Input: part model. Units: mm. Frame: model coordinates. A direction names the side the tool comes from. Coordinates: 2 decimals unless noted, no trailing zeros. Write each loop counter-clockwise with the first axis right and the second up, starting at its lowest first coordinate (ties: lowest second). Pieces come first, ordered by that corner, then holes. Notation, with made-up numbers: (81.5, 50) - (122.5, 50) arc R26 cw to (122.5, 68) - close; hole circle Ø1 at (40, 47.25). An arc over 180 degrees is marked (long way). Use a Markdown table: item, result. Add a question column.
Q1. Section query B-B (y = 0). Return the cut outline in (x, z).
Q2. Section query C-C (z = 17.7). Return the cut outline in (x, y).
Q3. Set-up query: faces 4 (the face through (36.198, 11.399, 80.98)), 5 (the face through (0.22, 41.258, 79.855)). Return all of +Z, -Z, +X, -X, +Y, -Y with unobstructed straight access to the full face (end or side cutting, diameter ignored); none if empty.
Q4. Material intervals for probe 1 along Z at (x, y) = (0, 40); probe 2 along Z at (x, y) = (7.5, -33.5); probe 3 along Y at (x, z) = (0, 62), sorted ascending. Write a range as from..to.
Q5. Mould query, pull axis X, two halves, no side actions, for faces 1 (the face through (-24, -30, 150)), 2 (the face through (0.22, -41.361, 79.855)), 3 (the face through (20.765, -39.923, 73.95)). Classes: released by +X, released by -X, zero draft, split by the parting line, or undercut.
Q6. Section query D-D (x = -16.5). Return the cut outline in (y, z).
Q7. Pin query (flat end, axial travel): P1, Ø3, axis at y = -16.5, z = 38.5, coming from the +X side; P2, Ø1.5, axis at y = -19.5, z = 58, coming from the +X side; P3, Ø5, axis at x = -20.5, z = 109.5, coming from the +Y side. Return the tip coordinate at first contact, or that it passes through.
Q8. Section query A-A (x = 0). Return the cut outline in (y, z), then the cut area to 4 significant figures.
from build123d import *

# Parameters (mm, degrees)
SKETCH1_R               = 45
BOSS_EXTRUDE1_DEPTH     = 150
SKETCH2_R               = 31.85
CUT_EXTRUDE1_DEPTH      = 163.941707368
SKETCH3_R               = 37.95
CUT_EXTRUDE2_DEPTH      = 140
CUT_EXTRUDE5_DEPTH      = 163.941707368
CUT_EXTRUDE5_DEPTH_BACK = 163.941707368
SKETCH8_R               = 5


with BuildPart() as part:
    # Sketch1 → Boss-Extrude1 (new body)
    with BuildSketch(Plane.XY):
        Circle(SKETCH1_R)
    extrude(amount=BOSS_EXTRUDE1_DEPTH)

    # Sketch2 → Cut-Extrude1 (cut, through all)
    with BuildSketch(Plane.XY.offset(150)):
        Circle(SKETCH2_R)
    extrude(amount=-CUT_EXTRUDE1_DEPTH, mode=Mode.SUBTRACT)

    # Sketch3 → Cut-Extrude2 (cut)
    with BuildSketch(Plane.XY.offset(150)):
        Circle(SKETCH3_R)
    extrude(amount=-CUT_EXTRUDE2_DEPTH, mode=Mode.SUBTRACT)

    # Sketch8 → Cut-Extrude5 (cut, two sides: drawn at the far end of the back side and taken through both)
    with BuildSketch(Plane(origin=(0, 0, 0), x_dir=(1, 0, 0), z_dir=(0, 1, 0)).offset(-CUT_EXTRUDE5_DEPTH_BACK)):
        with Locations(Location((0, -17.7, 0), (0, 0, 270))):
            Circle(SKETCH8_R)
        with Locations(Location((0, -84.85, 0), (0, 0, 270))):
            Circle(SKETCH8_R)
    extrude(amount=CUT_EXTRUDE5_DEPTH + CUT_EXTRUDE5_DEPTH_BACK, mode=Mode.SUBTRACT)


solid = part.part
Values follow:
| question | item | result |
|---|---|---|
| 1 | outline | (-45, 0) - (-31.85, 0) - (-31.85, 10) - (-37.95, 10) - (-37.95, 150) - (-45, 150) - close; (31.85, 0) - (45, 0) - (45, 150) - (37.95, 150) - (37.95, 10) - (31.85, 10) - close |
| 2 | outline | (-5, -44.72) - (-5, -37.62) arc R37.95 cw to (-5, 37.62) - (-5, 44.72) arc R45 ccw to start; (5, -44.72) arc R45 ccw to (5, 44.72) - (5, 37.62) arc R37.95 cw to (5, -37.62) - close |
| 3 | face 4 | +Z |
| 3 | face 5 | +Y, -Y |
| 4 | probe 1 | 0..12.7, 22.7..79.85, 89.85..150 |
| 4 | probe 2 | 0..10 |
| 4 | probe 3 | -45..-37.95, 37.95..45 |
| 5 | face 1 | zero draft |
| 5 | face 2 | undercut |
| 5 | face 3 | split by the parting line |
| 6 | outline | (-41.87, 0) - (-27.24, 0) - (-27.24, 10) - (-34.18, 10) - (-34.18, 150) - (-41.87, 150) - close; (27.24, 0) - (41.87, 0) - (41.87, 150) - (34.18, 150) - (34.18, 10) - (27.24, 10) - close |
| 7 | P1 | x = 42.43 |
| 7 | P2 | x = 40.91 |
| 7 | P3 | y = 41.24 |
| 8 | outline | (-45, 0) - (-31.85, 0) - (-31.85, 10) - (-37.95, 10) - (-37.95, 12.7) - (-45, 12.7) - close; (-45, 22.7) - (-37.95, 22.7) - (-37.95, 79.85) - (-45, 79.85) - close; (-45, 89.85) - (-37.95, 89.85) - (-37.95, 150) - (-45, 150) - close; (31.85, 0) - (45, 0) - (45, 12.7) - (37.95, 12.7) - (37.95, 10) - (31.85, 10) - close; (37.95, 22.7) - (45, 22.7) - (45, 79.85) - (37.95, 79.85) - close; (37.95, 89.85) - (45, 89.85) - (45, 150) - (37.95, 150) - close |
| 8 | area | 1,955 mm2 |
